Autodesk Inventor part; units mm, degrees
ref_plane "Work Plane1" through (0, -90, 0) normal (0, 1, 0) x (-1, 0, 0)
ref_plane "Work Plane2" through (-3, 20, 0) normal (0, 0, 1) x (1, 0, 0)
ref_plane "YZ Plane" through (0, 0, 0) normal (1, 0, 0) x (0, 1, 0)
sketch "Sketch1" plane through (0, 0, 0) normal (0, 0, 1) x (1, 0, 0)
  line L0 (0, 20) -> (0, 0)
  line L1 (0, 0) -> (50, 8.8163)
  arc A0 (50, 8.8163) -> (58.1206, 15.6304) centre (48.1592, 19.256) ccw
  line L2 (0, 0) -> (58.1206, 0) construction
  line L3 (58.1206, 15.6304) -> (52.4316, 0) construction
  line L4 (0, 20) -> (-3, 20)
  line L5 (-3, 20) -> (-3, -4.5907)
  line L6 (-3, -4.5907) -> (50.6946, 4.8771)
  arc A1 (50.6946, 4.8771) -> (61.8794, 14.2623) centre (48.1592, 19.256) ccw
  arc A2 (61.8794, 14.2623) -> (58.1206, 15.6304) centre (60, 14.9463) ccw
  dimension "d1" = 20
  dimension "d2" = 50
  dimension "d3" = 3
  dimension "d4" = 70
  dimension "d5" = 2
  dimension "d6" = 10
  dimension "d7" = 10
extrude "Extrusion1" add sketch "Sketch1" along normal mid plane 40
sketch "Sketch2" plane through (0, 0, 0) normal (0, 1, 0) x (-1, 0, 0)
  line L0 (3, 7) -> (-32, 7)
  line L1 (-32, 7) -> (-32, -7)
  line L2 (-32, -7) -> (3, -7)
  line L3 (3, -7) -> (3, 7)
  line L4 (3, -20) -> (3, 20)
  point P0 (0, 0)
  point P1 (3, 0)
  point P2 (3, 0)
  dimension "d10" = 14
  dimension "d11" = 35
extrude "Extrusion2" cut sketch "Sketch2" along normal through all both and the other way through all
ref_plane "Work Plane1" through (0, -90, 0) normal (0, 1, 0) x (-1, 0, 0)
sketch "Sketch3" plane through (0, -90, 0) normal (0, 1, 0) x (-1, 0, 0)
  line L0 (-60, -8.25) -> (-35, -8.25)
  line L1 (-35, -8.25) -> (-35, 8.25)
  line L2 (-35, 8.25) -> (-60, 8.25)
  line L3 (-60, 8.25) -> (-60, -8.25)
  line L4 (-60, -8.25) -> (-35, 8.25) construction
  line L5 (-35, -8.25) -> (-60, 8.25) construction
  line L6 (-32, -7) -> (-32, 7)
  point P0 (0, 0)
  point P1 (-47.5, 0)
  dimension "d27" = 25
  dimension "d28" = 16.5
  dimension "d29" = 3
extrude "Extrusion3" add sketch "Sketch3" along normal up to next
sketch "Sketch5" plane through (42, -90, 0) normal (0, -1, 0) x (1, 0, 0)
  line L0 (15.5, 5) -> (-4.5, 5)
  line L1 (-4.5, 5) -> (-4.5, -5)
  line L2 (-4.5, -5) -> (15.5, -5)
  line L3 (15.5, -5) -> (15.5, 5)
  line L4 (15.5, 5) -> (-4.5, -5) construction
  line L5 (-4.5, 5) -> (15.5, -5) construction
  line L6 (-7, 8.25) -> (18, 8.25)
  line L7 (18, 8.25) -> (18, -8.25)
  point P0 (-42, 0)
  point P1 (5.5, 0)
  point P2 (5.5, 8.25)
  point P3 (5.5, 5)
  point P4 (18, 0)
  point P5 (15.5, 0)
  dimension "d30" = 20
  dimension "d31" = 10
extrude "Extrusion4" cut sketch "Sketch5" against normal up to surface surface through (-3, -4.5907, 0) normal (0.1736482, -0.9848078, 0)
ref_plane "Work Plane2" through (-3, 20, 0) normal (0, 0, 1) x (1, 0, 0)
sketch "Sketch7" plane through (32, 1.5808, -7) normal (-1, 0, 0) x (0, 0, 1)
  line L0 (0, -7.9383) -> (14, -7.9383)
  line L1 (14, -7.9383) -> (14, 2.0617)
  line L2 (14, 2.0617) -> (0, 2.0617)
  line L3 (0, 2.0617) -> (0, -7.9383)
  line L4 (0, -7.9383) -> (14, 2.0617) construction
  line L5 (14, -7.9383) -> (0, 2.0617) construction
  line L6 (0, 4.0617) -> (14, 4.0617)
  point P0 (7, -1.5808)
  point P1 (7, -2.9383)
  point P2 (7, 4.0617)
  point P3 (7, 2.0617)
  dimension "d32" = 10
  dimension "d33" = 14
  dimension "d34" = 2
extrude "Extrusion5" cut sketch "Sketch7" against normal up to surface (25.5 mm away)
sketch "Sketch8" plane through (35, -90, 8.25) normal (0, 0, 1) x (1, 0, 0)
  line L0 (7.5, 4) -> (17.5, 4)
  line L1 (17.5, 4) -> (17.5, 0)
  line L2 (17.5, 0) -> (7.5, 0)
  line L3 (7.5, 0) -> (7.5, 4)
  line L4 (7.5, 4) -> (17.5, 0) construction
  line L5 (17.5, 4) -> (7.5, 0) construction
  line L6 (0, 0) -> (25, 0)
  point P0 (-35, 90)
  point P1 (12.5, 2)
  point P2 (12.5, 0)
  point P3 (12.5, 0)
  dimension "d37" = 10
  dimension "d38" = 4
extrude "Extrusion6" add sketch "Sketch8" along normal blind 10
sketch "Sketch9" plane through (42.5, -86, 8.25) normal (0, 1, 0) x (1, 0, 0)
  circle A0 centre (5, -5) radius 1.65
  circle A1 centre (5, -5) radius 3
  line L0 (10, 0) -> (10, -10)
  line L1 (10, -10) -> (0, -10)
  point P0 (-42.5, 8.25)
  point P1 (10, -5)
  point P2 (5, -10)
  dimension "d41" = 3.3
  dimension "d42" = 6
extrude "Extrusion7" cut sketch "Sketch9" against normal through all contours A0
extrude "Extrusion8" cut sketch "Sketch9" against normal blind 1.5
fillet "Fillet1" radius 2 4 edges at (52.5, -88, 18.25) (42.5, -88, 18.25) (52.5, -88, 8.25) (42.5, -88, 8.25)
mirror "Mirror1" about plane through (0, 0, 0) normal (0, 0, 1) of "Extrusion6", "Extrusion7", "Extrusion8", "Fillet1"
fillet_without_effect "Fillet2"
properties part number "Inclined Ramp"
The model under review builds one solid part; all positions refer to its coordinate system, in mm. A direction names the side the tool comes from. Round coordinates to 2 decimals unless told otherwise and drop trailing zeros. Loops run counter-clockwise (first coordinate to the right, second up) from the corner with the lowest first, then second, coordinate; pieces in that order, holes last. Notation, with made-up numbers: M 59,15.25 L 69,15.25 A23 cw 69,24.25 Z; hole C 67.25,52.5 d6. An arc over 180 degrees is marked long. Answer as CSV lines item,"result". Start each with the question number.
Item 1: Mouldability with a two-part tool opening along Y and no side actions: class faces 1 (the face through (25, 4, -20)), 2 (the face through (43.7, -6.358, -5.2)), 3 (the face through (55.033, 11.186, -0.28)) as released by +Y, released by -Y, zero draft, split by the parting line, or undercut.
Item 2: Consider section D-D (x = 18). Write out the cut boundary in (y, z).
Item 3: Consider section B-B (y = -79). Write out the cut boundary in (x, z), then the cut area to 4 significant figures.
Item 4: For faces 4 (the face through (44.503, -86.74, -13.382)), 5 (the face through (52.5, -88, -13)), 6 (the face through (48, -88, -18.25)), 7 (the face through (39, 3.642, 0)), 8 (the face through (52, 4, -5)), list the 3-axis set-ups (+Z, -Z, +X, -X, +Y, -Y) from which the entire face can be reached by the end or side of a thin tool; tool diameter is ignored.
Item 5: Wall thickness on line 1 (Z direction, x = 47.5, y = -86.95); line 2 (Z direction, x = 47.5, y = -88.9); line 3 (Z direction, x = 39, y = -49): over which ranges is each line inside the solid? List them lowest first. Write a range as [from, to].
Item 6: Consider section A-A (z = 13.25). Write out the cut boundary in (x, y), then the cut area to 3 significant figures.
Item 7: Consider section C-C (x = 7). Write out the cut boundary in (y, z), then the cut area to 3 significant figures.
Item 8: Insertion check: P1, Ø12, axis at y = -44, z = 9, coming from the +X side; P2, Ø2, axis at y = -22, z = 1, coming from the -X side; P3, Ø8, axis at x = 49.5, z = 8.5, coming from the +Y side. Each pin has a flat end and moves straight along its axis. Give the tip position at first contact, or say it passes through.
Answer:
1,face 1,"zero draft"
1,face 2,"undercut"
1,face 3,"released by +Y"
2,outline,"M -0.89,-20 L 3.17,-20 L 3.17,-7 L -0.89,-7 Z; M -0.89,7 L 3.17,7 L 3.17,20 L -0.89,20 Z"
3,outline,"M 35,-8.25 L 60,-8.25 L 60,8.25 L 35,8.25 Z; hole M 37.5,-5 L 57.5,-5 L 57.5,5 L 37.5,5 Z"
3,area,"212.5 mm^2"
4,face 4,"none"
4,face 5,"-Z, +X, -Y"
4,face 6,"-Z, +X, -X, -Y"
4,face 7,"-X"
4,face 8,"-Y"
5,line 1,"z = [-18.25, -16.25], [-10.25, -5], [5, 10.25], [16.25, 18.25]"
5,line 2,"z = [-18.25, -14.9], [-11.6, -5], [5, 11.6], [14.9, 18.25]"
5,line 3,"z = [-8.25, -5], [5, 8.25]"
6,outline,"M -3,-4.59 L 50.69,4.88 A14.6 ccw 61.88,14.26 A2 ccw 58.12,15.63 A10.6 cw 50,8.82 L 0,0 L 0,20 L -3,20 Z; M 42.5,-90 L 45.85,-90 L 45.85,-87.5 L 44.5,-87.5 L 44.5,-86 L 42.5,-86 Z; M 49.15,-90 L 52.5,-90 L 52.5,-86 L 50.5,-86 L 50.5,-87.5 L 49.15,-87.5 Z"
6,area,"359 mm^2"
7,outline,"M -2.83,-20 L 1.23,-20 L 1.23,-7 L -2.83,-7 Z; M -2.83,7 L 1.23,7 L 1.23,20 L -2.83,20 Z"
7,area,"106 mm^2"
8,P1,"stops at x = 60"
8,P2,"stops at x = 35"
8,P3,"stops at y = 10.1"
